Can you work these out from the drawing? Everything is in mm from the part's minimum corner. Round coordinates to 2 decimals unless told otherwise and drop trailing zeros. Write each loop counter-clockwise with the first axis right and the second up, starting at its lowest first coordinate (ties: lowest second). Pieces come first, ordered by that corner, then holes. Notation, with made-up numbers: M -25,56 L 26,56 A12 cw 26,78 Z; hole C 7,65 d9. An arc over 180 degrees is marked long. Use one line per item in the form item = value. Start each with the question number.
Q1. I need wall thicknesses on line 1 along X through (y, z) = (18.5, 13.5); line 2 along Z through (x, y) = (267.5, 49). Which ranges of each line are inside material? Lowest first, please. Write a range as from..to.
Q2. We'd pull the mould along X, two halves only. Please class the marked faces 1, 2 and 3: +X half, -X half, draft (parallel to the pull), parting line (faces both ways), or undercut.
Q3. I'm going to push a flat-ended pin straight in: pin 1 Ø10 at (x, z) = (59.5, 55) entering from -Y. Where does the tip first touch, or does it pass through?
Q4. I want a section at C-C on y = 45. List the corners of the cut face in (x, z) for me, and give its area (3 significant figures).
Q5. I want a section at B-B on y = 61. List the corners of the cut face in (x, z) for me, and give its area (3 significant figures).
Q6. I want a section at A-A on z = 70.5. List the corners of the cut face in (x, y) for me.
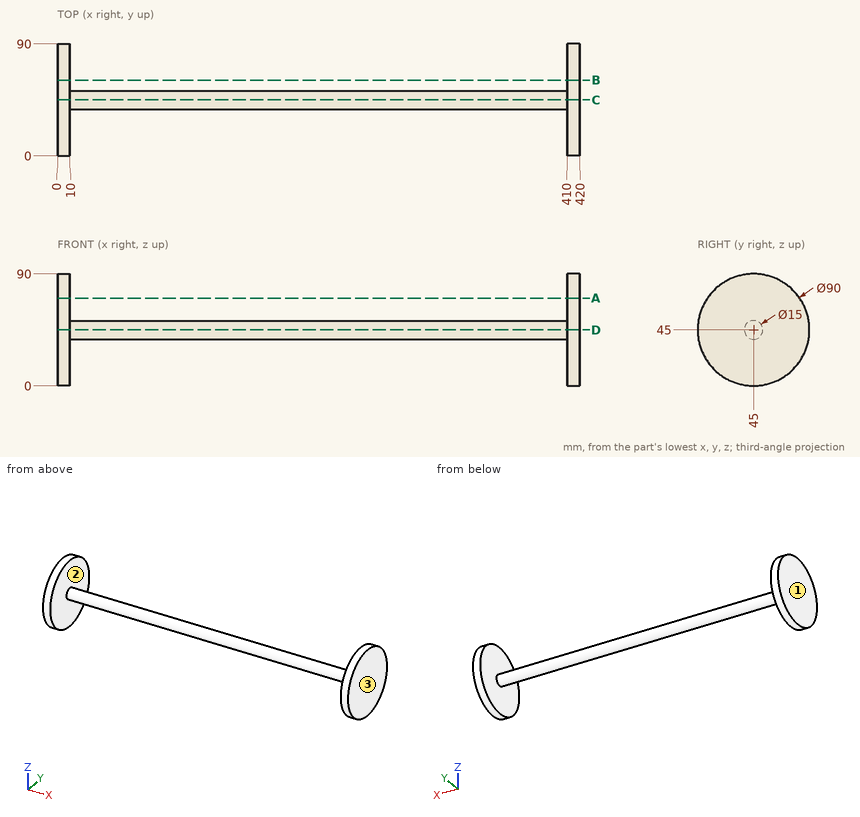
Reported:
q1.line_1 = 0..10, 410..420
q1.line_2 = 38.66..51.34
q2.face_1 = -X half
q2.face_2 = undercut
q2.face_3 = +X half
q3.pin_1 = 39.41
q4.outline = M 0,0 L 10,0 L 10,37.5 L 410,37.5 L 410,0 L 420,0 L 420,90 L 410,90 L 410,52.5 L 10,52.5 L 10,90 L 0,90 Z
q4.area = 7,800 mm^2
q5.outline = M 0,2.94 L 10,2.94 L 10,87.06 L 0,87.06 Z; M 410,2.94 L 420,2.94 L 420,87.06 L 410,87.06 Z
q5.area = 1,680 mm^2
q6.outline = M 0,7.92 L 10,7.92 L 10,82.08 L 0,82.08 Z; M 410,7.92 L 420,7.92 L 420,82.08 L 410,82.08 Z
